Part model, mm, in its own coordinate system. Face numbers are marked on the shaded views. A direction names the side the tool comes from. Round coordinates to 2 decimals unless told otherwise and drop trailing zeros. Write each loop counter-clockwise with the first axis right and the second up, starting at its lowest first coordinate (ties: lowest second). Pieces come first, ordered by that corner, then holes.
1) Saw through at B-B on y = 9. Write the cut outline in (x, z), and give its area (3 significant figures).
2) Pull direction Z, two halves, no side cores. Call the marked faces 1 and 2: +Z half, -Z half, draft (parallel to the pull), parting line (faces both ways), or undercut.
3) Saw through at C-C on x = 10. Write the cut outline in (y, z), and give its area (3 significant figures).
4) Drill centre lines: L1, parallel to Z at x = 0, y = 1.9; L2, parallel to Y at x = 0, z = -17.2; L3, parallel to Y at x = 13, z = -3.5. Where is each one in solid material? Low to high.
5) Saw through at D-D on y = 31. Write the cut outline in (x, z), and give its area (3 significant figures).
6) Which spindle directions (+Z, -Z, +X, -X, +Y, -Y) get a long thin tool onto all of the face, cutting with end or side? Do the marked faces 3 and 4. Say none if no direction does.
7) Flat gauge pins, fed straight in: pin 1 (4 mm diameter, centred on x = 0, z = 0, fed in from +Y); pin 2 (8 mm diameter, centred on y = 28, z = 9.5, fed in from -X); pin 3 (10 mm diameter, centred on x = 14.5, y = 13.5, fed in from -Z); pin 4 (2 mm diameter, centred on x = 7.5, y = 10, fed in from -Z). Where does each tip first touch, or does it go through?
8) Saw through at A-A on z = 0. Write the cut outline in (x, y).
Autodesk Inventor part; units mm, degrees
ref_plane "YZ Plane" through (0, 0, 0) normal (1, 0, 0) x (0, 1, 0)
ref_plane "XZ Plane" through (0, 0, 0) normal (0, 1, 0) x (-1, 0, 0)
ref_plane "XY Plane" through (0, 0, 0) normal (0, 0, 1) x (1, 0, 0)
sketch "Sketch1" plane through (0, 0, 0) normal (0, 1, 0) x (-1, 0, 0)
  circle A0 centre (0, 0) radius 20
  dimension "d0" = 40
extrude "Extrusion1" add sketch "Sketch1" along normal blind 5
sketch "Sketch2" plane through (0, 5, 0) normal (0, 1, 0) x (1, 0, 0)
  circle A0 centre (0, 0) radius 20
  line L0 (-12, 16) -> (12, 16)
  line L1 (-12, -16) -> (12, -16)
  dimension "d3" = 4
  dimension "d4" = 4
extrude "Extrusion2" add sketch "Sketch2" along normal blind 30 contours L0 A0 | A0 L1
sketch "Sketch4" plane through (12, 5, 16) normal (0, 0, -1) x (-1, 0, 0)
  line L0 (24, 30) -> (24, 17.9)
  line L1 (0, 30) -> (0, 17.9)
  arc A0 (11.8923, 29.9) -> (0, 17.9) centre (12, 17.9005) ccw
  arc A1 (24, 17.9) -> (11.8923, 29.9) centre (12, 17.9005) ccw
  line L2 (0, 30) -> (24, 30)
  point P0 (12, -5)
  dimension "d10" = 12.1
  dimension "d11" = 12.1
  dimension "d12" = 12
  dimension "d13" = 12
extrude "Extrusion3" cut sketch "Sketch4" against normal blind 25
sketch "Sketch5" plane through (-12, 5, -16) normal (0, 0, 1) x (1, 0, 0)
  line L0 (24, 30) -> (24, 17.9)
  line L1 (0, 30) -> (0, 17.9)
  arc A0 (12, 29.9) -> (0, 17.9) centre (12, 17.9) ccw
  arc A1 (24, 17.9) -> (12, 29.9) centre (12, 17.9) ccw
  line L2 (24, 30) -> (0, 30)
  line L3 (0, 30) -> (24, 30)
  point P0 (12, -5)
  dimension "d16" = 12.1
  dimension "d17" = 12.1
  dimension "d18" = 12
  dimension "d19" = 12
extrude "Extrusion4" cut sketch "Sketch5" against normal blind 25
sketch "Sketch6" plane through (-12, 5, -16) normal (0, 0, 1) x (1, 0, 0)
  circle A0 centre (12, 18.8433) radius 1.5
  line L0 (0, 0) -> (0, 18.8433)
  line L1 (0, 18.8433) -> (23.891, 18.8433)
  point P0 (12, -5)
  dimension "d22" = 3
  dimension "d23" = 12
  dimension "d24" = 0
extrude "Extrusion5" cut sketch "Sketch6" along normal mid plane 500
fillet "Fillet1" radius 2 2 edges at (0, 5, 16) (0, 5, -16)
sketch "Sketch7" plane through (0, 5, 0) normal (0, 1, 0) x (1, 0, 0)
  circle A0 centre (0, 0) radius 1.5
  dimension "d28" = 3
extrude "Extrusion6" cut sketch "Sketch7" against normal blind 10
properties part number "hlava"
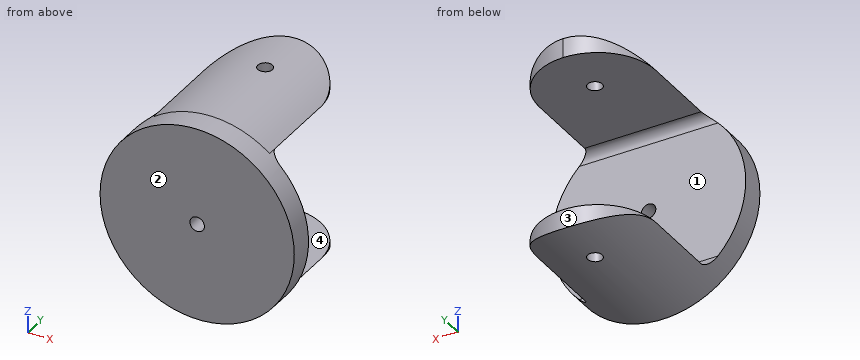
Completed:
1. outline: (-12, -16) arc R20 ccw to (12, -16) - close; (-12, 16) - (12, 16) arc R20 ccw to start
1. area: 131 mm2
2. face 1: undercut
2. face 2: draft
3. outline: (0, -17.32) - (29.53, -17.32) - (29.53, -16) - (7, -16) arc R2 cw to (5, -14) - (5, 14) arc R2 cw to (7, 16) - (29.53, 16) - (29.53, 17.32) - (0, 17.32) - close
3. area: 240 mm2
4. L1: z = -20 to -1.5, 1.5 to 20
4. L2: y = 0 to 22.34, 25.34 to 34.9
4. L3: y = 0 to 5
5. outline: (-8.85, -17.93) arc R20 ccw to (8.85, -17.93) - (8.85, -16) - (-8.85, -16) - close; (-8.85, 16) - (8.85, 16) - (8.85, 17.93) arc R20 ccw to (-8.85, 17.93) - close
5. area: 118 mm2
6. face 3: +Z, -Z, +Y
6. face 4: +X, -X, +Y
7. pin 1: stops at y = 5
7. pin 2: passes through
7. pin 3: stops at z = -17.6
7. pin 4: stops at z = -18.91
8. outline: (-20, 0) - (-1.5, 0) - (-1.5, 5) - (-20, 5) - close; (1.5, 0) - (20, 0) - (20, 5) - (1.5, 5) - close
